from build123d import *

# Parameters (mm, degrees)
SKETCH1_W               = 96.131545064
SKETCH1_H               = 62
BOSS_EXTRUDE1_DEPTH     = 3.175
SKETCH2_W               = 96.131545064
SKETCH2_H               = 1
EXTRUDE_THIN1_DEPTH     = 33.175
LPATTERN1_COUNT         = 19
LPATTERN1_PITCH         = 3.388888889
CUT_EXTRUDE1_DEPTH      = 67.120338127
CUT_EXTRUDE1_DEPTH_BACK = 67.120338127


with BuildPart() as part:
    # Sketch1 → Boss-Extrude1 (new body)
    with BuildSketch(Plane(origin=(0, 0, 0), x_dir=(0, 0, -1), z_dir=(1, 0, 0))):
        Rectangle(SKETCH1_W, SKETCH1_H)
    extrude(amount=BOSS_EXTRUDE1_DEPTH)

    # Sketch2 → Extrude-Thin1 (add)
    with BuildSketch(Plane(origin=(3.175, 0, 0), x_dir=(0, 0, -1), z_dir=(1, 0, 0))):
        with Locations((0, 30.5)):
            Rectangle(SKETCH2_W, SKETCH2_H)
    extrude_thin1 = extrude(amount=EXTRUDE_THIN1_DEPTH)

    # LPattern1: Extrude-Thin1 ×19
    with Locations(*[(0, -i * LPATTERN1_PITCH, 0) for i in range(1, LPATTERN1_COUNT)]):
        add(extrude_thin1)

    # Sketch3 → Cut-Extrude1 (cut, two sides: drawn at the far end of the back side and taken through both)
    with BuildSketch(Plane(origin=(3.175, 0, 0), x_dir=(0, 0, -1), z_dir=(1, 0, 0)).offset(-CUT_EXTRUDE1_DEPTH_BACK)):
        Polygon((-0.096506061, -46.331819287), (-55.483661094, 9.055335745), (-88.096831181, -23.557834342), (-32.709676149, -78.944989375), align=None)
    extrude(amount=CUT_EXTRUDE1_DEPTH + CUT_EXTRUDE1_DEPTH_BACK, mode=Mode.SUBTRACT)


solid = part.part
Work out the finished part from the listing and answer in its coordinate system (mm). A direction names the side the tool comes from. Coordinates: 2 decimals unless noted, no trailing zeros. Order: outer loops, then holes, each group sorted by start corner. A loop starts at its lowest first (then second) coordinate and runs counter-clockwise, first axis right, second up. Notation, with made-up numbers: (80, 65) - (134, 65) arc R27 ccw to (134, 83) - close; hole circle Ø4 at (-22, -28.75). An arc over 180 degrees is marked (long way). Put each result on its own line as item: value. Start each with the question number.
1) For faces 3 (the flat face through (14, 17, 48.066)), 4 (the flat face through (3.175, -19, -9)), determine the directions among +Z, -Z, +X, -X, +Y, -Y from which every point of the face is accessible in a straight line to the end or side of a thin tool.
2) Find section B-B (y = 22). Give the vertices of the cut face in (x, z) (3 decimals), plus the area to 3 significant figures.
3) Flat-ended cylindrical pins translate along their axes: pin 1 (1 mm diameter, centred on x = 28.5, z = 35.5, fed in from -Y); pin 2 (2.5 mm diameter, centred on y = -18, z = 5.5, fed in from +X); pin 3 (3 mm diameter, centred on x = 12, y = -7.5, fed in from +Z); pin 4 (0.7 mm diameter, centred on y = -29, z = -18.5, fed in from +X) (3 decimals). Find the tip coordinate at first contact, or state that the pin passes through.
4) Find the intervals of material crossed by line 1 (X direction, y = -15.5, z = -33) (3 decimals); line 2 (Z direction, x = 15, y = -3.5); line 3 (Z direction, x = 32, y = 0), in increasing order. Write a range as from..to.
5) Find section C-C (y = -5). Give the vertices of the cut face in (x, z) (3 decimals), plus the area to 3 significant figures.
6) Find section A-A (x = 23.5). State how many separate pieces and enclosed holes the cut face has, plus the area to 3 significant figures.
7) For a pull along Y with two mould halves and no side action, classify faces 1 (the flat face through (20, 7.278, 1)), 2 (the flat face through (0, 0, 1)) as released by +Y, released by -Y, zero draft, split by the parting line, or undercut.
Results list:
1. face 3: +Z, +X, -X, +Y, -Y
1. face 4: +Z, -Z, +X
2. outline: (0, -48.066) - (3.175, -48.066) - (3.175, 48.066) - (0, 48.066) - close
2. area: 305 mm^2
3. pin 1: stops at y = -10.67
3. pin 2: stops at x = 36.35
3. pin 3: stops at z = 40.15
3. pin 4: stops at x = 3.175
4. line 1: x = 0..3.175
4. line 2: z = -48.07..42.93
4. line 3: z = -48.07..46.43
5. outline: (0, -48.066) - (3.175, -48.066) - (3.175, 41.428) - (0, 41.428) - close
5. area: 284 mm^2
6. separate pieces: 19
6. enclosed holes: 0
6. area: 1,660 mm^2
7. face 1: undercut
7. face 2: zero draft
